```python
from build123d import *

# Parameters (mm, degrees)
IZIM1_R                     = 167.5
IZIM1_R_2                   = 148
Y_KSEKLIK_EKSTR_ZYON2_DEPTH = 185.3
IZIM9_R                     = 3.4
KES_EKSTR_ZYON1_DEPTH       = 15
IZIM10_W                    = 5
IZIM10_H                    = 16.407796145
Y_KSEKLIK_EKSTR_ZYON3_DEPTH = 180
IZIM13_W                    = 308.627991419
IZIM13_H                    = 53.891387346
KES_EKSTR_ZYON2_DEPTH       = 333
IZIM12_R                    = 5
KES_EKSTR_ZYON3_DEPTH       = 333


with BuildPart() as part:
    # Çizim1 → Yükseklik-Ekstrüzyon2 (new body)
    with BuildSketch(Plane.XY):
        Circle(IZIM1_R)
        Circle(IZIM1_R_2, mode=Mode.SUBTRACT)
    extrude(amount=Y_KSEKLIK_EKSTR_ZYON2_DEPTH)

    # Çizim9 → Kes-Ekstrüzyon1 (cut)
    with BuildSketch(Plane(origin=(0, 0, 0), x_dir=(-1, 0, 0), z_dir=(0, 0, -1))):
        with Locations((107.349895203, -112.5)):
            Circle(IZIM9_R)
        with Locations((-107.349895203, -112.5)):
            Circle(IZIM9_R)
        with Locations((-107.349895203, 112.5)):
            Circle(IZIM9_R)
        with Locations((107.349895203, 112.5)):
            Circle(IZIM9_R)
    kes_ekstr_zyon1 = extrude(amount=-KES_EKSTR_ZYON1_DEPTH, mode=Mode.SUBTRACT)

    # Çizim10 → Döndür1 (revolve)
    with BuildSketch(Plane(origin=(0, 0, 0), x_dir=(0, 0, -1), z_dir=(1, 0, 0)), mode=Mode.PRIVATE) as d_nd_r1_sk:
        with Locations((-32.5, 150.703898073)):
            Rectangle(IZIM10_W, IZIM10_H)
    revolve(d_nd_r1_sk.sketch.rotate(Axis((0, 0, 0), (0, 0, 1)), 90), axis=Axis((0, 0, 0), (0, 0, 1)))

    # Aynalama1: Kes-Ekstrüzyon1 across plane
    add(kes_ekstr_zyon1.mirror(Plane(origin=(0, 0, 92.65), x_dir=(1, 0, 0), z_dir=(0, 0, -1))), mode=Mode.SUBTRACT)


with BuildPart() as body_2:
    # Çizim11 → Yükseklik-Ekstrüzyon3 (new body)
    with BuildSketch(Plane.XY):
        with BuildLine():
            Line((120, -116.859958925), (120, -200))
            Line((120, -200), (-120, -200))
            Line((-120, -200), (-120, -116.859958925))
            ThreePointArc((-120, -116.859958925), (0, -167.5), (120, -116.859958925))
        make_face()
    extrude(amount=Y_KSEKLIK_EKSTR_ZYON3_DEPTH)

    # Çizim13 → Kes-Ekstrüzyon2 (cut)
    with BuildSketch(Plane.XY.offset(180)):
        with Locations((-6.112680509, -223.805652598)):
            Rectangle(IZIM13_W, IZIM13_H)
    extrude(amount=-KES_EKSTR_ZYON2_DEPTH, mode=Mode.SUBTRACT)

    # Çizim12 → Kes-Ekstrüzyon3 (cut)
    with BuildSketch(Plane.XZ.offset(200)):
        with Locations((-75, 152.5)):
            Circle(IZIM12_R)
        with Locations((75, 152.5)):
            Circle(IZIM12_R)
        with Locations((75, 27.5)):
            Circle(IZIM12_R)
        with Locations((-75, 27.5)):
            Circle(IZIM12_R)
    extrude(amount=-KES_EKSTR_ZYON3_DEPTH, mode=Mode.SUBTRACT)


solid = body_2.part
```
Read the model definition and answer for the solid it produces. Units are mm, in the model's axes. Give positions to 0.01 mm unless a question says otherwise; leave off trailing zeros. Loops run counter-clockwise (first coordinate to the right, second up) from the corner with the lowest first, then second, coordinate; pieces in that order, holes last.
Item 1: The part is cut by section A-A (y = -165). Write down the section's boundary in (x, z), and give its area (3 significant figures).
Item 2: The mould has two halves that part along X. Classify faces 1 (the cylindrical face through (-79.995, -172.339, 152.72)), 2 (the flat face through (2, -174, 180)), 3 (the flat face through (120, -156, 89)), 4 (the flat face through (-120, -157, 89)): released by +X, released by -X, zero draft, split by the parting line, or undercut.
Item 3: The part is cut by section B-B (z = 27.5). Write down the section's boundary in (x, y), and give its area (3 significant figures).
Item 4: Find the intervals of material crossed by line 1 along Z through (x, y) = (75, -180); line 2 along X through (y, z) = (-183, 152.5); line 3 along X through (y, z) = (-180, 25), in increasing order.
Item 5: The part is cut by section D-D (x = 75). Write down the section's boundary in (y, z), and give its area (3 significant figures).
Item 6: Each of these flat-tipped pins is pushed along its axis until it touches: pin 1 Ø8 at (x, z) = (75, 27.5) entering from -Y; pin 2 Ø8 at (x, z) = (-26.5, 154.5) entering from +Y; pin 3 Ø16 at (x, z) = (75, 152.5) entering from +Y; pin 4 Ø13 at (x, z) = (-75, 152.5) entering from +Y. Where does it stop, or does it pass through?
Item 7: The part is cut by section C-C (y = -132.5). Write down the section's boundary in (x, z), and give its area (3 significant figures).
Taken from the geometry:
1. outline: (-120, 0) - (-28.83, 0) - (-28.83, 180) - (-120, 180) - close; (28.83, 0) - (120, 0) - (120, 180) - (28.83, 180) - close; hole circle Ø10 at (-75, 27.5); hole circle Ø10 at (-75, 152.5); hole circle Ø10 at (75, 27.5); hole circle Ø10 at (75, 152.5)
1. area: 32,500 mm2
2. face 1: undercut
2. face 2: zero draft
2. face 3: released by +X
2. face 4: released by -X
3. outline: (-120, -196.86) - (-80, -196.86) - (-80, -147.16) arc R167.5 cw to (-120, -116.86) - close; (-70, -196.86) - (70, -196.86) - (70, -152.17) arc R167.5 cw to (-70, -152.17) - close; (80, -196.86) - (120, -196.86) - (120, -116.86) arc R167.5 cw to (80, -147.16) - close
3. area: 9,870 mm2
4. line 1: z = 0 to 22.5, 32.5 to 147.5, 157.5 to 180
4. line 2: x = -120 to -80, -70 to 70, 80 to 120
4. line 3: x = -120 to -79.33, -70.67 to 70.67, 79.33 to 120
5. outline: (-196.86, 0) - (-149.77, 0) - (-149.77, 22.5) - (-196.86, 22.5) - close; (-196.86, 32.5) - (-149.77, 32.5) - (-149.77, 147.5) - (-196.86, 147.5) - close; (-196.86, 157.5) - (-149.77, 157.5) - (-149.77, 180) - (-196.86, 180) - close
5. area: 7,530 mm2
6. pin 1: passes through
6. pin 2: stops at y = -164.7
6. pin 3: stops at y = -145.49
6. pin 4: stops at y = -146.34
7. outline: (-120, 0) - (-102.47, 0) - (-102.47, 180) - (-120, 180) - close; (102.47, 0) - (120, 0) - (120, 180) - (102.47, 180) - close
7. area: 6,310 mm2
